Source: CAD feature listing. Evaluate the final solid. Frame: model axes, mm. A direction names the side the tool comes from. Round coordinates to 2 decimals unless told otherwise and drop trailing zeros. Write each loop counter-clockwise with the first axis right and the second up, starting at its lowest first coordinate (ties: lowest second). Pieces come first, ordered by that corner, then holes. Notation, with made-up numbers: M 28,-15 L 36,-15 A16 cw 36,14 Z; hole C -15,-22.75 d2. An arc over 180 degrees is marked long. Use a Markdown table: item, result.
```python
from build123d import *

# Parameters (mm, degrees)
SKETCH029_W             = 9
SKETCH029_H             = 3
PAD012_DEPTH            = 2.5
SKETCH030_R             = 1.55
PAD013_DEPTH            = 2.2
SKETCH035_W             = 9
SKETCH035_H             = 0.75
PAD014_DEPTH            = 3
SKETCH036_W             = 6
SKETCH036_H             = 0.75
PAD015_DEPTH            = 3
SKETCH037_W             = 6
SKETCH037_H             = 0.75
PAD016_DEPTH            = 3
SKETCH048_W             = 15
SKETCH048_H             = 0.75
PAD022_DEPTH            = 1.5
SKETCH049_W             = 2.255218
SKETCH049_H             = 8.498976
POCKET022_DEPTH         = 1
BODY003_PLACEMENT_ANGLE = 90


with BuildPart() as part:
    # Sketch029 → Pad012 (new body)
    with BuildSketch(Plane.XZ):
        with Locations((10.557257, 18.562511)):
            Rectangle(SKETCH029_W, SKETCH029_H)
    extrude(amount=PAD012_DEPTH)

    # Sketch030 (on Face6 of Pad012) → Pad013 (join)
    with BuildSketch(Plane.XZ.offset(2.5)):
        with Locations((10.557257, 18.562511)):
            Circle(SKETCH030_R)
    extrude(amount=PAD013_DEPTH)

    # Sketch035 → Pad014 (join)
    with BuildSketch(Plane(origin=(0, 0, 17.062511), x_dir=(1, 0, 0), z_dir=(0, 0, -1))):
        with Locations((10.557257, 0.375)):
            Rectangle(SKETCH035_W, SKETCH035_H)
    extrude(amount=PAD014_DEPTH)

    # Sketch036 (on Face15 of Pad014) → Pad015 (join)
    with BuildSketch(Plane(origin=(15.057257, 0, 0), x_dir=(0, 0, 1), z_dir=(1, 0, 0))):
        with Locations((17.062511, 0.375)):
            Rectangle(SKETCH036_W, SKETCH036_H)
    extrude(amount=PAD015_DEPTH)

    # Sketch037 (on Face3 of Pad015) → Pad016 (join)
    with BuildSketch(Plane(origin=(6.057257, 0, 0), x_dir=(0, 0, -1), z_dir=(-1, 0, 0))):
        with Locations((-17.062511, 0.375)):
            Rectangle(SKETCH037_W, SKETCH037_H)
    extrude(amount=PAD016_DEPTH)

    # Sketch048 (on Face5 of Pad016) → Pad022 (join)
    with BuildSketch(Plane(origin=(0, 0, 20.062511), x_dir=(-1, 0, 0), z_dir=(0, 0, 1))):
        with Locations((-10.557257, 0.375)):
            Rectangle(SKETCH048_W, SKETCH048_H)
    extrude(amount=PAD022_DEPTH)

    # Sketch049 (on Face23 of Pad022) → Pocket022 (cut)
    with BuildSketch(Plane(origin=(0, 0, 0), x_dir=(1, 0, 0), z_dir=(0, 1, 0))):
        with Locations((10.556244, -17.71185)):
            Rectangle(SKETCH049_W, SKETCH049_H)
    extrude(amount=-POCKET022_DEPTH, mode=Mode.SUBTRACT)


with BuildPart() as part_1:
    # Body003 placement: moved
    add(part.part.moved(Location((146.5, 10.6, 9.6))).rotate(Axis((146.5, 10.6, 9.6), (1, 0, 0)), BODY003_PLACEMENT_ANGLE))


solid = part_1.part
```
Q1. Section D-D on x = 156.5. Return loops of the section in (y, z).
Results are:
| item | result |
|---|---|
| outline | M -9.46,7.1 L -9.41,7.1 L -9.41,4.9 L -6.52,4.9 L -6.52,7.1 L -6.46,7.1 L -6.46,8.6 L -9.46,8.6 Z |
Q2. Section A-A on y = -10.25. Return loops of the section in (x, z).
Results are:
| item | result |
|---|---|
| outline | M 149.56,8.85 L 155.93,8.85 L 155.93,9.6 L 149.56,9.6 Z; M 158.18,8.85 L 164.56,8.85 L 164.56,9.6 L 158.18,9.6 Z |
Q3. Section C-C on y = -7.75. Return loops of the section in (x, z), plus the area to 3 significant figures.
Results are:
| item | result |
|---|---|
| outline | M 149.56,8.85 L 152.56,8.85 L 152.56,7.1 L 155.52,7.1 L 155.52,4.9 L 158.59,4.9 L 158.59,7.1 L 161.56,7.1 L 161.56,8.85 L 164.56,8.85 L 164.56,9.6 L 158.18,9.6 L 158.18,8.6 L 155.93,8.6 L 155.93,9.6 L 149.56,9.6 Z |
| area | 31.5 mm^2 |
Q4. Section B-B on x = 160. Return loops of the section in (y, z).
Results are:
| item | result |
|---|---|
| outline | M -10.96,8.85 L -9.46,8.85 L -9.46,7.1 L -6.46,7.1 L -6.46,8.85 L -3.46,8.85 L -3.46,9.6 L -10.96,9.6 Z |
Q5. Mould query, pull axis X, two halves, no side actions, for faces 5 (the flat face through (155.929, -7, 9)), 6 (the flat face through (157, -8, 8.6)), 7 (the flat face through (153, -7, 9.6)), 8 (the flat face through (161.557, -8, 8)). Classes: +X half, -X half, draft (parallel to the pull), parting line (faces both ways), or undercut.
Results are:
| item | result |
|---|---|
| face 5 | undercut |
| face 6 | undercut |
| face 7 | draft |
| face 8 | +X half |
Q6. First-contact query: pin 1 Ø1.9 at (x, y) = (153, -6.5) entering from -Z; pin 2 Ø0.5 at (x, z) = (155.5, 7.5) entering from -Y; pin 3 Ø1.8 at (x, y) = (157, -7.5) entering from +Z. Flat tips, straight axial feed; report the tip coordinate or a pass-through.
Results are:
| item | result |
|---|---|
| pin 1 | z = 7.1 |
| pin 2 | y = -9.46 |
| pin 3 | z = 8.6 |
Q7. Line query: L1, parallel to X at y = -7.5, z = 8.9; L2, parallel to X at y = -6.75, z = 7.85; L3, parallel to Y at x = 153.5, z = 7.3. Output: solid intervals per line, ascending.
Results are:
| item | result |
|---|---|
| L1 | 149.56 to 155.93, 158.18 to 164.56 |
| L2 | 152.56 to 161.56 |
| L3 | -9.46 to -6.46 |
Q8. Reachability of faces 1 (the flat face through (161, -7, 9.6)), 2 (the flat face through (152.557, -8, 8)), 3 (the flat face through (158.184, -7, 9)), 4 (the cylindrical face through (155.51, -8.03, 6.02)) from +Z, -Z, +X, -X, +Y, -Y: full face, straight path, thin tool, end or side. Return the list, or none.
Results are:
| item | result |
|---|---|
| face 1 | +Z, +X, -X, +Y, -Y |
| face 2 | -Z, -X, +Y, -Y |
| face 3 | +Z, +Y, -Y |
| face 4 | -Z |
